Input: part model. Units: mm. Frame: model coordinates. A direction names the side the tool comes from. Coordinates: 2 decimals unless noted, no trailing zeros. Write each loop counter-clockwise with the first axis right and the second up, starting at its lowest first coordinate (ties: lowest second). Pieces come first, ordered by that corner, then holes.
1) Set-up query: faces 4 (the flat face through (0, -86, -65.775)), 5 (the cylindrical face through (17.9, -7.8, -80.3)), 6 (the cylindrical face through (-0.46, -74.18, -43.45)), 7 (the flat face through (0, -86, -70.725)), 8 (the flat face through (0, -86, -20.275)). Return all of +Z, -Z, +X, -X, +Y, -Y with unobstructed straight access to the full face (end or side cutting, diameter ignored); none if empty.
2) Draft query along X for faces 1 (the conical face through (0.079, -64.557, -80.506)), 2 (the conical face through (12.11, -89.865, -68.204)), 3 (the flat face through (21, 0, -45)). Return one class per face: pulls with the +X half, pulls with the -X half, needs draft (parallel to the pull), parting line crosses it, or undercut.
3) Section query C-C (z = -22.75). Output: boundary loops of the cut face in (x, y) (3 decimals), then the cut area to 3 significant figures.
4) Line query: L1, parallel to Z at x = 0, y = -72.5; L2, parallel to X at y = -7.75, z = -45.5; L3, parallel to Z at x = 20, y = -5. Output: solid intervals per line, ascending.
5) Pin query (flat end, axial travel): pin 1 Ø1 at (x, z) = (-2.5, -38.5) entering from +Y; pin 2 Ø4.5 at (x, y) = (-5.5, -10.5) entering from +Z; pin 3 Ø3 at (y, z) = (-45, -44) entering from -X; pin 4 Ø5 at (x, z) = (-20, -80.25) entering from -Y. Return the tip coordinate at first contact, or that it passes through.
6) Section query A-A (z = -68.25). Output: boundary loops of the cut face in (x, y) (3 decimals).
7) Section query B-B (y = -44). Output: boundary loops of the cut face in (x, z), then the cut area to 3 significant figures.
from build123d import *

# Parameters (mm, degrees)
BOSS_EXTRUDE1_DEPTH = 91
SKETCH8_W           = 3
SKETCH8_H           = 9.5
SKETCH8_H_2         = 18.5
M5X0_81_REACH       = 127.678
M5X0_81_BORE_R      = 2.1
BOSS_EXTRUDE2_DEPTH = 7
CHAMFER1_SIZE       = 0.5
CHAMFER_1_SIZE      = 1
M5X0_82_D           = 4.2
M5X0_82_DEPTH       = 17.4
M5X0_82_TIP         = 1.2618073


with BuildPart() as part:
    # Sketch1 → Boss-Extrude1 (new body)
    with BuildSketch(Plane.XY):
        with BuildLine():
            Line((12, 0), (25, 0))
            Line((25, 0), (25, -10))
            Line((25, -10), (15, -18))
            Line((15, -18), (15, -65))
            Line((15, -65), (25, -73))
            Line((25, -73), (25, -83))
            Line((25, -83), (-25, -83))
            Line((-25, -83), (-25, -73))
            Line((-25, -73), (-15, -65))
            Line((-15, -65), (-15, -18))
            Line((-15, -18), (-25, -10))
            Line((-25, -10), (-25, 0))
            Line((-25, 0), (-12, 0))
            ThreePointArc((-12, 0), (0, -12), (12, 0))
        make_face()
    extrude(amount=-BOSS_EXTRUDE1_DEPTH)

    # Sketch8 → Cut-Revolve2 (revolve, cut)
    with BuildSketch(Plane(origin=(0, 0, 0), x_dir=(1, 0, 0), z_dir=(0, 1, 0))):
        with Locations((13.5, 80.25)):
            Rectangle(SKETCH8_W, SKETCH8_H)
        with Locations((13.5, 15.25)):
            Rectangle(SKETCH8_W, SKETCH8_H_2)
    revolve(axis=Axis((0, 0, -91), (0, 0, 1)), mode=Mode.SUBTRACT)

    # Отверстие обработанное метчиком M5x0.81 bore → Отверстие обработанное метчиком M5x0.81 (cut, up to next)
    with BuildSketch(Plane(origin=(0, 0, 0), x_dir=(1, 0, 0), z_dir=(0, 1, 0)), mode=Mode.PRIVATE) as m5x0_81_sk1:
        with Locations((-20, 10.75)):
            Circle(M5X0_81_BORE_R)
    m5x0_81_tool1 = extrude(m5x0_81_sk1.sketch, amount=-M5X0_81_REACH, mode=Mode.PRIVATE) & part.part
    # Отверстие обработанное метчиком M5x0.81 bore → Отверстие обработанное метчиком M5x0.81 (cut, up to next)
    with BuildSketch(Plane(origin=(0, 0, 0), x_dir=(1, 0, 0), z_dir=(0, 1, 0)), mode=Mode.PRIVATE) as m5x0_81_sk2:
        with Locations((20, 10.75)):
            Circle(M5X0_81_BORE_R)
    m5x0_81_tool2 = extrude(m5x0_81_sk2.sketch, amount=-M5X0_81_REACH, mode=Mode.PRIVATE) & part.part
    # Отверстие обработанное метчиком M5x0.81 bore → Отверстие обработанное метчиком M5x0.81 (cut, up to next)
    with BuildSketch(Plane(origin=(0, 0, 0), x_dir=(1, 0, 0), z_dir=(0, 1, 0)), mode=Mode.PRIVATE) as m5x0_81_sk3:
        with Locations((-20, 80.25)):
            Circle(M5X0_81_BORE_R)
    m5x0_81_tool3 = extrude(m5x0_81_sk3.sketch, amount=-M5X0_81_REACH, mode=Mode.PRIVATE) & part.part
    # Отверстие обработанное метчиком M5x0.81 bore → Отверстие обработанное метчиком M5x0.81 (cut, up to next)
    with BuildSketch(Plane(origin=(0, 0, 0), x_dir=(1, 0, 0), z_dir=(0, 1, 0)), mode=Mode.PRIVATE) as m5x0_81_sk4:
        with Locations((20, 80.25)):
            Circle(M5X0_81_BORE_R)
    m5x0_81_tool4 = extrude(m5x0_81_sk4.sketch, amount=-M5X0_81_REACH, mode=Mode.PRIVATE) & part.part
    # Отверстие обработанное метчиком M5x0.81 bore → Отверстие обработанное метчиком M5x0.81 (cut, up to next)
    with BuildSketch(Plane(origin=(0, 0, 0), x_dir=(1, 0, 0), z_dir=(0, 1, 0)), mode=Mode.PRIVATE) as m5x0_81_sk5:
        with Locations((-18.5, 45.5)):
            Circle(M5X0_81_BORE_R)
    m5x0_81_tool5 = extrude(m5x0_81_sk5.sketch, amount=-M5X0_81_REACH, mode=Mode.PRIVATE) & part.part
    # Отверстие обработанное метчиком M5x0.81 bore → Отверстие обработанное метчиком M5x0.81 (cut, up to next)
    with BuildSketch(Plane(origin=(0, 0, 0), x_dir=(1, 0, 0), z_dir=(0, 1, 0)), mode=Mode.PRIVATE) as m5x0_81_sk6:
        with Locations((18.5, 45.5)):
            Circle(M5X0_81_BORE_R)
    m5x0_81_tool6 = extrude(m5x0_81_sk6.sketch, amount=-M5X0_81_REACH, mode=Mode.PRIVATE) & part.part
    add(m5x0_81_tool1.solids().sort_by_distance((-20, 0, -10.75))[0], mode=Mode.SUBTRACT)
    add(m5x0_81_tool2.solids().sort_by_distance((20, 0, -10.75))[0], mode=Mode.SUBTRACT)
    add(m5x0_81_tool3.solids().sort_by_distance((-20, 0, -80.25))[0], mode=Mode.SUBTRACT)
    add(m5x0_81_tool4.solids().sort_by_distance((20, 0, -80.25))[0], mode=Mode.SUBTRACT)
    add(m5x0_81_tool5.solids().sort_by_distance((-18.5, 0, -45.5))[0], mode=Mode.SUBTRACT)
    add(m5x0_81_tool6.solids().sort_by_distance((18.5, 0, -45.5))[0], mode=Mode.SUBTRACT)

    # Sketch9 → Boss-Extrude2 (add)
    with BuildSketch(Plane.XZ.offset(83)):
        with BuildLine():
            Line((-10, -25.225), (10, -25.225))
            ThreePointArc((10, -25.225), (12.475, -22.75), (10, -20.275))
            Line((10, -20.275), (-10, -20.275))
            ThreePointArc((-10, -20.275), (-12.475, -22.75), (-10, -25.225))
        make_face()
        with BuildLine():
            Line((-10, -65.775), (10, -65.775))
            ThreePointArc((10, -65.775), (12.475, -68.25), (10, -70.725))
            Line((10, -70.725), (-10, -70.725))
            ThreePointArc((-10, -70.725), (-12.475, -68.25), (-10, -65.775))
        make_face()
    extrude(amount=BOSS_EXTRUDE2_DEPTH)

    # Chamfer1
    chamfer1_edges = [part.edges().sort_by_distance(p)[0] for p in [
        (12.475, -90, -22.75),
        (0, -90, -20.275),
        (-12.475, -90, -22.75),
        (0, -90, -25.225),
        (12.475, -90, -68.25),
        (0, -90, -65.775),
        (-12.475, -90, -68.25),
        (0, -90, -70.725),
    ]]
    chamfer(chamfer1_edges, length=CHAMFER1_SIZE)

    # Фаска1
    chamfer_1_edges = [part.edges().sort_by_distance(p)[0] for p in [
        (-25, 0, -45.5),
        (25, 0, -45.5),
    ]]
    chamfer(chamfer_1_edges, length=CHAMFER_1_SIZE)

    # Отверстие обработанное метчиком M5x0.82
    with Locations(Plane(origin=(0, -83, 0), x_dir=(-1, 0, 0), z_dir=(0, -1, 0))):
        with Locations((0, 45.5), (0, 10.1375), (0, 80.8625)):
            Hole(M5X0_82_D / 2, depth=M5X0_82_DEPTH)
            with Locations((0, 0, -(M5X0_82_DEPTH + M5X0_82_TIP / 2))):  # 118° drill point
                Cone(0, M5X0_82_D / 2, M5X0_82_TIP, mode=Mode.SUBTRACT)


solid = part.part
Answer:
1. face 4: +X, -X, -Y
1. face 5: +Y
1. face 6: -Y
1. face 7: -Z, +X, -X, -Y
1. face 8: +Z, +X, -X, -Y
2. face 1: undercut
2. face 2: pulls with the +X half
2. face 3: needs draft
3. outline: (-25, -83) - (-12.475, -83) - (-12.475, -89.5) - (-11.975, -90) - (11.975, -90) - (12.475, -89.5) - (12.475, -83) - (25, -83) - (25, -73) - (15, -65) - (15, -18) - (25, -10) - (25, -1) - (24, 0) - (15, 0) arc R15 cw to (-15, 0) - (-24, 0) - (-25, -1) - (-25, -10) - (-15, -18) - (-15, -65) - (-25, -73) - close
3. area: 2,870 mm2
4. L1: z = -91 to -82.96, -78.76 to -47.6, -43.4 to -12.24, -8.04 to 0
4. L2: x = -25 to -20.6, -16.4 to -9.16, 9.16 to 16.4, 20.6 to 25
4. L3: z = -91 to -82.35, -78.15 to -46.97, -44.03 to -12.85, -8.65 to 0
5. pin 1: stops at y = -11.62
5. pin 2: stops at z = 0
5. pin 3: stops at x = -15
5. pin 4: stops at y = -83
6. outline: (-25, -83) - (-12.475, -83) - (-12.475, -89.5) - (-11.975, -90) - (11.975, -90) - (12.475, -89.5) - (12.475, -83) - (25, -83) - (25, -73) - (15, -65) - (15, -18) - (25, -10) - (25, -1) - (24, 0) - (12, 0) arc R12 cw to (-12, 0) - (-24, 0) - (-25, -1) - (-25, -10) - (-15, -18) - (-15, -65) - (-25, -73) - close
7. outline: (-15, -91) - (15, -91) - (15, 0) - (-15, 0) - close
7. area: 2,730 mm2
